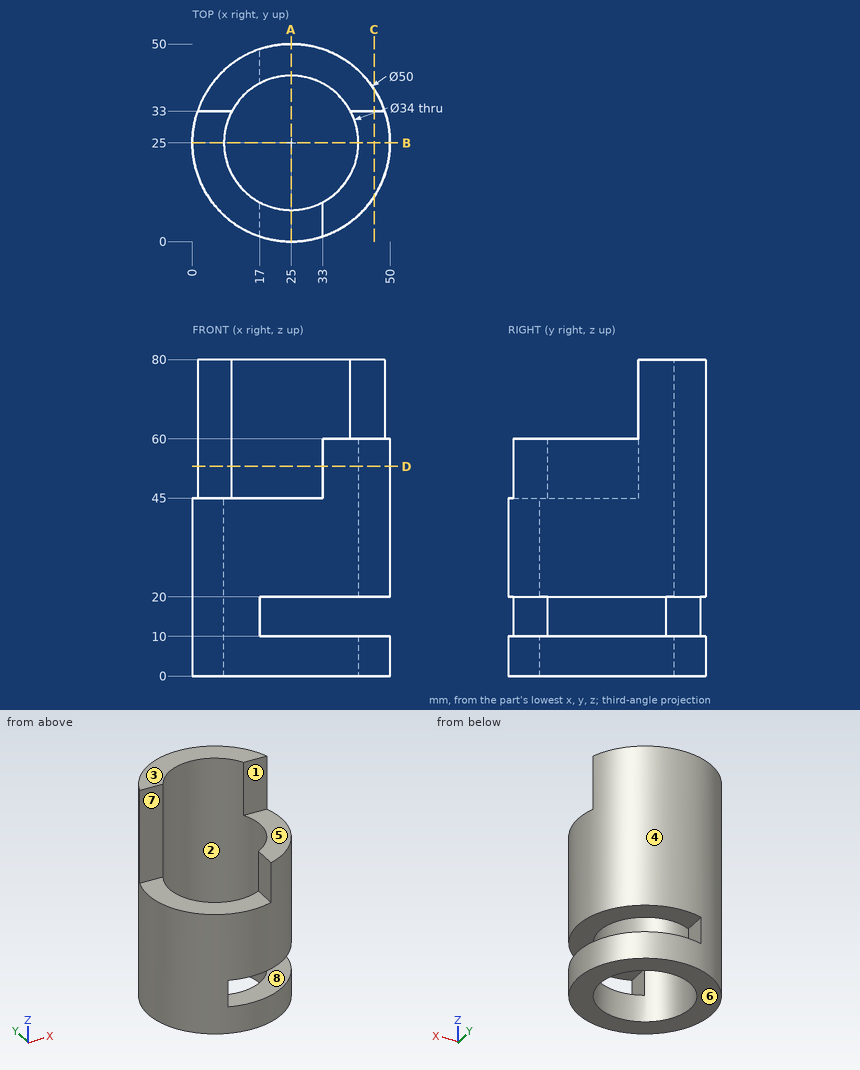
The drawing under review shows one solid part. Ordinate dimensions are in mm from its lowest x, y, z. A direction names the side the tool comes from. Give positions to 0.01 mm unless a question says otherwise; leave off trailing zeros. Loops run counter-clockwise (first coordinate to the right, second up) from the corner with the lowest first, then second, coordinate; pieces in that order, holes last. Notation, with made-up numbers: M 29,61 L 37,61 A31 cw 37,94 Z; hole C 41,6.25 d2. An arc over 180 degrees is marked long. Return JSON: item names as keys, results as strings. Group by question number.
Item 1: Insertion check: pin 1 Ø2.5 at (x, z) = (4, 67.5) entering from -Y; pin 2 Ø4.5 at (y, z) = (7, 12.5) entering from +X; pin 3 Ø1 at (y, z) = (7, 44) entering from -X; pin 4 Ø10 at (x, y) = (24.5, 15.5) entering from -Z. Each pin has a flat end and moves straight along its axis. Give the tip position at first contact, or say it passes through.
Item 2: Tool access review of the marked faces 5, 6, 7 and 8: name each direction out of +Z, -Z, +X, -X, +Y, -Y from which nothing blocks a thin tool from reaching the whole face with its end or side.
Item 3: We need section D-D (z = 53). Give the boundary of the cut face in (x, y), and give its area (3 significant figures).
Item 4: We need section B-B (y = 25). Give the boundary of the cut face in (x, z).
Item 5: For probe 1 along X at (y, z) = (25, 25); probe 2 along Z at (x, y) = (44, 20); probe 3 along Z at (x, y) = (36, 40.5), list the stretches that pass through material, from the lowest coordinate up.
Item 6: We need section C-C (x = 46). Give the boundary of the cut face in (y, z).
Item 7: We need section A-A (x = 25). Give the boundary of the cut face in (y, z).
Item 8: Mouldability with a two-part tool opening along Y and no side actions: class the marked faces 1, 2, 3 and 4 as released by +Y, released by -Y, zero draft, split by the parting line, or undercut.
Output:
{
 "1": {"pin 1": "stops at y = 33", "pin 2": "stops at x = 17", "pin 3": "stops at x = 7.15", "pin 4": "passes through"},
 "2": {"face 5": "+Z, +X, -X, -Y", "face 6": "-Z, +X, -X, +Y, -Y", "face 7": "+Z, -X, -Y", "face 8": "+X, +Y, -Y"},
 "3": {"outline": "M 1.31,33 L 10,33 A17 cw long 33,10 L 33,1.31 A25 ccw long Z", "area": "660 mm^2"},
 "4": {"outline": "M 0,0 L 8,0 L 8,45 L 0,45 Z; M 42,0 L 50,0 L 50,10 L 42,10 Z; M 42,20 L 50,20 L 50,60 L 42,60 Z"},
 "5": {"probe 1": "x = 0 to 8, 42 to 50", "probe 2": "z = 0 to 10, 20 to 60", "probe 3": "z = 0 to 10, 20 to 80"},
 "6": {"outline": "M 11.44,0 L 38.56,0 L 38.56,10 L 11.44,10 Z; M 11.44,20 L 38.56,20 L 38.56,80 L 33,80 L 33,60 L 11.44,60 Z"},
 "7": {"outline": "M 0,0 L 8,0 L 8,10 L 0,10 Z; M 0,20 L 8,20 L 8,45 L 0,45 Z; M 42,0 L 50,0 L 50,10 L 42,10 Z; M 42,20 L 50,20 L 50,80 L 42,80 Z"},
 "8": {"face 1": "released by -Y", "face 2": "undercut", "face 3": "zero draft", "face 4": "split by the parting line"}
}
